Read the model definition and answer for the solid it produces. Units are mm, in the model's axes. Give positions to 0.01 mm unless a question says otherwise; leave off trailing zeros. Loops run counter-clockwise (first coordinate to the right, second up) from the corner with the lowest first, then second, coordinate; pieces in that order, holes last. Notation, with made-up numbers: (67.5, 67.25) - (119.5, 67.25) arc R30 ccw to (119.5, 102.25) - close; hole circle Ø4 at (76.5, 83.25). An arc over 180 degrees is marked (long way). Write each question's results on one line, items separated by ' | '. Start each with the question number.
Q1. The part is cut by section B-B, the plane z = -19.5. Write down the section's boundary in (x, y), plus the area to 3 significant figures.
Q2. Find the intervals of material crossed by line 1 (X direction, y = 3.5, z = -61); line 2 (X direction, y = -64, z = -39); line 3 (Z direction, x = -87.5, y = -1), in increasing order. Write a range as from..to.
Q3. The part is cut by section C-C, the plane z = -65.5. Write down the section's boundary in (x, y).
Q4. The part is cut by section D-D, the plane x = 28. Write down the section's boundary in (y, z), plus the area to 3 significant figures.
Q5. Given pin 1 (5 mm diameter, centred on y = 24, z = -105, fed in from +X); pin 2 (1 mm diameter, centred on y = -32, z = -57, fed in from +X); pin 3 (5 mm diameter, centred on x = -12, y = 16, fed in from +Z), each flat-ended and moving along its own axis, determine where each tip first touches the part or whether it passes through.
Q6. Determine the mould class of faces 1 (the flat face through (16.285, -0.805, -71.59)), 2 (the flat face through (-1, -1, -173.205)), 3 (the flat face through (-14.376, -0.805, -63.101)), 4 (the flat face through (-1, 75, -105)) for opening direction Y: +Y half, -Y half, draft (parallel to the pull), parting line (faces both ways), or undercut.
```python
from build123d import *

# Parameters (mm, degrees)
F1_DEPTH = 75
F2_R     = 10
F3_DEPTH = 150.001
F4_W     = 26
F4_H     = 70.1128626734
F5_DEPTH = 44


with BuildPart() as f1:
    # F0 (on Front) → F1 (new body, symmetric)
    with BuildSketch(Plane.XZ):
        Polygon((100, -173.2050807569), (0, 0), (-100, -173.2050807569), align=None)
    extrude(amount=F1_DEPTH, both=True)

    # F2 (on face) → F3 (cut, through all)
    with BuildSketch(Plane(origin=(0, 75, 0), x_dir=(-1, 0, 0), z_dir=(0, 1, 0))):
        with Locations((-7.4031245895, -38.9061681926)):
            Circle(F2_R)
    extrude(amount=-F3_DEPTH, mode=Mode.SUBTRACT)

    # F4 (on face) → F5 (cut)
    with BuildSketch(Plane(origin=(0, 0, 0), x_dir=(0, 1, 0), z_dir=(0.8660254038, 0, 0.5))):
        with Locations((-0.6230119616, -35.0847196241)):
            Rectangle(F4_W, F4_H)
    extrude(amount=-F5_DEPTH, mode=Mode.SUBTRACT)


solid = f1.part
```
Check sheet entries:
1) outline: (-11.26, -75) - (11.26, -75) - (11.26, -13.62) - (-11.26, -13.62) - close; (-11.26, 12.38) - (11.26, 12.38) - (11.26, 75) - (-11.26, 75) - close | area: 2,790 mm^2
2) line 1: x = -35.22..-15.59, 34.63..35.22 | line 2: x = -22.52..-2.6, 17.4..22.52 | line 3: z = -173.21..-151.55
3) outline: (-37.82, -75) - (37.82, -75) - (37.82, 75) - (-37.82, 75) - close; hole (-12.99, -13.62) - (26.83, -13.62) - (26.83, 12.38) - (-12.99, 12.38) - close
4) outline: (-75, -173.21) - (75, -173.21) - (75, -48.5) - (12.38, -48.5) - (12.38, -64.83) - (-13.62, -64.83) - (-13.62, -48.5) - (-75, -48.5) - close | area: 18,300 mm^2
5) pin 1: stops at x = 62.07 | pin 2: stops at x = 33.2 | pin 3: stops at z = -16.45
6) face 1: undercut | face 2: draft | face 3: undercut | face 4: +Y half
